```python
from build123d import *

# Parameters (mm, degrees)
SKETCH_1_W           = 270
SKETCH_1_H           = 250
SKETCH_1_R           = 1.55
EXTRUDE_1_DEPTH      = 3
SKETCH_2_R           = 40
CUT_EXTRUDE_1_DEPTH  = 10
CUT_EXTRUDE_3_DEPTH  = 10
SKETCH_5_R           = 5
SKETCH_5_R_2         = 1.55
CUT_EXTRUDE_4_DEPTH  = 10
SKETCH_6_R           = 42.5
CUT_EXTRUDE_5_DEPTH  = 10
SKETCH_8_W           = 100
SKETCH_8_H           = 70
CUT_EXTRUDE_7_DEPTH  = 10
SKETCH_9_R           = 1.55
CUT_EXTRUDE_8_DEPTH  = 10
SKETCH_10_R          = 1.55
CUT_EXTRUDE_9_DEPTH  = 10
SKETCH_11_R          = 1.55
CUT_EXTRUDE_10_DEPTH = 10
FILLET_3_R           = 8
SKETCH_13_W          = 34
SKETCH_13_H          = 48
SKETCH_13_W_2        = 7
SKETCH_13_H_2        = 7
SKETCH_13_R          = 1.55
CUT_EXTRUDE_12_DEPTH = 10
FILLET_4_R           = 1.5
SKETCH_15_R          = 1.55
CUT_EXTRUDE_13_DEPTH = 10
SKETCH_16_R          = 4.05
CUT_EXTRUDE_14_DEPTH = 10
CUT_EXTRUDE_START    = -10
SKETCH_19_R          = 4.05
CUT_EXTRUDE_19_DEPTH = 10
SKETCH_21_R          = 1.55
CUT_EXTRUDE_20_DEPTH = 10
SKETCH_23_W          = 7
SKETCH_23_H          = 19
CUT_EXTRUDE_22_DEPTH = 10
FILLET_8_R           = 2
SKETCH_12_W          = 2
SKETCH_12_H          = 35.6
SKETCH_12_R          = 1.1
CUT_EXTRUDE_23_DEPTH = 10
FILLET_9_R           = 5
SKETCH_26_R          = 1.55
CUT_EXTRUDE_24_DEPTH = 8


with BuildPart() as part:
    # 草图1 → 凸台-拉伸1 (new body)
    with BuildSketch(Plane(origin=(0, 0, 0), x_dir=(1, 0, 0), z_dir=(0, 1, 0))):
        Rectangle(SKETCH_1_W, SKETCH_1_H)
        with Locations(Location((132, 72, 0), (0, 0, 270))):
            Circle(SKETCH_1_R, mode=Mode.SUBTRACT)
        with Locations(Location((132, -72, 0), (0, 0, 270))):
            Circle(SKETCH_1_R, mode=Mode.SUBTRACT)
    extrude(amount=EXTRUDE_1_DEPTH)

    # 草图2 → 切除-拉伸1 (cut)
    with BuildSketch(Plane(origin=(0, 3, 0), x_dir=(1, 0, 0), z_dir=(0, 1, 0))):
        with Locations((-3, -95)):
            Circle(SKETCH_2_R)
    extrude(amount=-CUT_EXTRUDE_1_DEPTH, mode=Mode.SUBTRACT)

    # 草图4 → 切除-拉伸3 (cut)
    with BuildSketch(Plane(origin=(0, 3, 0), x_dir=(1, 0, 0), z_dir=(0, 1, 0))):
        Polygon((-90, -125), (-135, -70), (-162.976707817, -172.035264534), align=None)
        Polygon((-90, 125), (-135, 70), (-171.69806915, 153.777299788), align=None)
    extrude(amount=-CUT_EXTRUDE_3_DEPTH, mode=Mode.SUBTRACT)

    # 草图5 → 切除-拉伸4 (cut)
    with BuildSketch(Plane(origin=(0, 3, 0), x_dir=(1, 0, 0), z_dir=(0, 1, 0))):
        with Locations(Location((-87.852813742, 75, 0), (0, 0, 270))):
            Circle(SKETCH_5_R)
        with Locations(Location((-3, 95, 0), (0, 0, 270))):
            Circle(SKETCH_5_R)
        with Locations(Location((81.852813742, 75, 0), (0, 0, 270))):
            Circle(SKETCH_5_R)
        with Locations(Location((-87.852813742, 90, 0), (0, 0, 270))):
            Circle(SKETCH_5_R_2)
        with Locations(Location((-74.862432686, 67.5, 0), (0, 0, 270))):
            Circle(SKETCH_5_R_2)
        with Locations(Location((-100.843194799, 67.5, 0), (0, 0, 270))):
            Circle(SKETCH_5_R_2)
        with Locations(Location((-3, 110, 0), (0, 0, 270))):
            Circle(SKETCH_5_R_2)
        with Locations(Location((9.990381057, 87.5, 0), (0, 0, 270))):
            Circle(SKETCH_5_R_2)
        with Locations(Location((-15.990381057, 87.5, 0), (0, 0, 270))):
            Circle(SKETCH_5_R_2)
        with Locations(Location((81.852813742, 90, 0), (0, 0, 270))):
            Circle(SKETCH_5_R_2)
        with Locations(Location((94.843194799, 67.5, 0), (0, 0, 270))):
            Circle(SKETCH_5_R_2)
        with Locations(Location((68.862432686, 67.5, 0), (0, 0, 270))):
            Circle(SKETCH_5_R_2)
    extrude(amount=-CUT_EXTRUDE_4_DEPTH, mode=Mode.SUBTRACT)

    # 草图6 → 切除-拉伸5 (cut)
    with BuildSketch(Plane(origin=(0, 3, 0), x_dir=(1, 0, 0), z_dir=(0, 1, 0))):
        with Locations((-3, -95)):
            Circle(SKETCH_6_R)
    extrude(amount=-CUT_EXTRUDE_5_DEPTH, mode=Mode.SUBTRACT)

    # 草图8 → 切除-拉伸7 (cut)
    with BuildSketch(Plane(origin=(0, 3, 0), x_dir=(1, 0, 0), z_dir=(0, 1, 0))):
        with Locations((135, 0)):
            Rectangle(SKETCH_8_W, SKETCH_8_H)
    extrude(amount=-CUT_EXTRUDE_7_DEPTH, mode=Mode.SUBTRACT)

    # 草图9 → 切除-拉伸8 (cut)
    with BuildSketch(Plane(origin=(0, 3, 0), x_dir=(1, 0, 0), z_dir=(0, 1, 0))):
        with Locations(Location((-52.5, 67, 0), (0, 0, 270))):
            Circle(SKETCH_9_R)
    extrude(amount=-CUT_EXTRUDE_8_DEPTH, mode=Mode.SUBTRACT)

    # 草图10 → 切除-拉伸9 (cut)
    with BuildSketch(Plane(origin=(0, 3, 0), x_dir=(1, 0, 0), z_dir=(0, 1, 0))):
        with Locations(Location((57, 103, 0), (0, 0, 270))):
            Circle(SKETCH_10_R)
    extrude(amount=-CUT_EXTRUDE_9_DEPTH, mode=Mode.SUBTRACT)

    # 草图11 → 切除-拉伸10 (cut)
    with BuildSketch(Plane(origin=(0, 3, 0), x_dir=(1, 0, 0), z_dir=(0, 1, 0))):
        with Locations(Location((-52.5, -39, 0), (0, 0, 270))):
            Circle(SKETCH_11_R)
    extrude(amount=-CUT_EXTRUDE_10_DEPTH, mode=Mode.SUBTRACT)

    # 圆角3
    fillet_3_edges = [part.edges().sort_by_distance(p)[0] for p in [
        (135, 1.5, 35),
        (135, 1.5, -35),
        (85, 1.5, 35),
        (85, 1.5, -35),
        (-135, 1.5, -70),
        (-135, 1.5, 70),
        (-90, 1.5, -125),
        (135, 1.5, 125),
        (135, 1.5, -125),
    ]]
    fillet(fillet_3_edges, radius=FILLET_3_R)

    # 草图13 → 切除-拉伸12 (cut)
    with BuildSketch(Plane(origin=(0, 3, 0), x_dir=(1, 0, 0), z_dir=(0, 1, 0))):
        with Locations((10, 26)):
            Rectangle(SKETCH_13_W, SKETCH_13_H)
        with Locations((30.5, 26)):
            Rectangle(SKETCH_13_W_2, SKETCH_13_H)
        with Locations((10, 53.5)):
            Rectangle(SKETCH_13_W, SKETCH_13_H_2)
        with Locations((-10.5, 26)):
            Rectangle(SKETCH_13_W_2, SKETCH_13_H)
        with Locations((10, -1.5)):
            Rectangle(SKETCH_13_W, SKETCH_13_H_2)
        with Locations(Location((30, 0, 0), (0, 0, 270))):
            Circle(SKETCH_13_R)
        with Locations(Location((-10, 52, 0), (0, 0, 270))):
            Circle(SKETCH_13_R)
        with Locations(Location((-10, 0, 0), (0, 0, 270))):
            Circle(SKETCH_13_R)
        with Locations(Location((30, 52, 0), (0, 0, 270))):
            Circle(SKETCH_13_R)
    extrude(amount=-CUT_EXTRUDE_12_DEPTH, mode=Mode.SUBTRACT)

    # 圆角4
    fillet_4_edges = [part.edges().sort_by_distance(p)[0] for p in [
        (-7, 1.5, -2),
        (-14, 1.5, -2),
        (-14, 1.5, -50),
        (-7, 1.5, -50),
        (-7, 1.5, -57),
        (27, 1.5, -57),
        (27, 1.5, -50),
        (34, 1.5, -50),
        (34, 1.5, -2),
        (27, 1.5, -2),
        (27, 1.5, 5),
        (-7, 1.5, 5),
    ]]
    fillet(fillet_4_edges, radius=FILLET_4_R)

    # 草图15 → 切除-拉伸13 (cut)
    with BuildSketch(Plane(origin=(0, 3, 0), x_dir=(1, 0, 0), z_dir=(0, 1, 0))):
        with Locations(Location((47.5, -105, 0), (0, 0, 270))):
            Circle(SKETCH_15_R)
        with Locations(Location((-52.5, -105, 0), (0, 0, 270))):
            Circle(SKETCH_15_R)
        with Locations(Location((47.5, -57, 0), (0, 0, 270))):
            Circle(SKETCH_15_R)
        with Locations(Location((-52.5, -57, 0), (0, 0, 270))):
            Circle(SKETCH_15_R)
    extrude(amount=-CUT_EXTRUDE_13_DEPTH, mode=Mode.SUBTRACT)

    # 草图16 → 切除-拉伸14 (cut)
    with BuildSketch(Plane.XZ):
        with Locations(Location((-53, -105, 0), (0, 0, 270))):
            Circle(SKETCH_16_R)
    extrude(amount=-CUT_EXTRUDE_14_DEPTH, mode=Mode.SUBTRACT)

    # 草图19 → 切除-拉伸19 (cut)
    with BuildSketch(Plane(origin=(0, 3, 0), x_dir=(1, 0, 0), z_dir=(0, 1, 0)).offset(CUT_EXTRUDE_START)):
        with Locations(Location((-53, 105, 0), (0, 0, 90))):
            Circle(SKETCH_19_R)
        with Locations(Location((47, 105, 0), (0, 0, 270))):
            Circle(SKETCH_19_R)
    extrude(amount=CUT_EXTRUDE_19_DEPTH, mode=Mode.SUBTRACT)

    # 草图21 → 切除-拉伸20 (cut)
    with BuildSketch(Plane(origin=(0, 0, 0), x_dir=(-1, 0, 0), z_dir=(0, -1, 0))):
        with Locations(Location((-132.26, -117.45, 0), (0, 0, 90))):
            Circle(SKETCH_21_R)
        with Locations(Location((-70.88, -117.45, 0), (0, 0, 90))):
            Circle(SKETCH_21_R)
        with Locations(Location((-70.88, -81.94, 0), (0, 0, 90))):
            Circle(SKETCH_21_R)
        with Locations(Location((-132.26, -81.94, 0), (0, 0, 90))):
            Circle(SKETCH_21_R)
    extrude(amount=-CUT_EXTRUDE_20_DEPTH, mode=Mode.SUBTRACT)

    # 草图23 → 切除-拉伸22 (cut)
    with BuildSketch(Plane(origin=(0, 0, 0), x_dir=(-1, 0, 0), z_dir=(0, -1, 0))):
        with Locations((-131.5, -94.44)):
            Rectangle(SKETCH_23_W, SKETCH_23_H)
    extrude(amount=-CUT_EXTRUDE_22_DEPTH, mode=Mode.SUBTRACT)

    # 圆角8
    fillet_8_edges = [part.edges().sort_by_distance(p)[0] for p in [
        (135, 1.5, 103.94),
        (135, 1.5, 84.94),
        (128, 1.5, 84.94),
        (128, 1.5, 103.94),
    ]]
    fillet(fillet_8_edges, radius=FILLET_8_R)

    # 草图12 → 切除-拉伸23 (cut)
    with BuildSketch(Plane(origin=(0, 3, 0), x_dir=(1, 0, 0), z_dir=(0, 1, 0))):
        with Locations((-113.775, 0)):
            Rectangle(SKETCH_12_W, SKETCH_12_H)
        with Locations((-111.775, 0)):
            Rectangle(SKETCH_12_W, SKETCH_12_H)
        Polygon((-73.975, 31.25), (-112.775, 31.25), (-112.775, 17.8), (-110.775, 17.8), (-110.775, -17.8), (-112.775, -17.8), (-112.775, -31.25), (-73.975, -31.25), align=None)
        with Locations(Location((-112.975, 34.2, 0), (0, 0, 270))):
            Circle(SKETCH_12_R)
        with Locations(Location((-73.975, 34.2, 0), (0, 0, 270))):
            Circle(SKETCH_12_R)
        with Locations(Location((-112.975, -34.2, 0), (0, 0, 270))):
            Circle(SKETCH_12_R)
        with Locations(Location((-73.975, -34.2, 0), (0, 0, 270))):
            Circle(SKETCH_12_R)
    extrude(amount=-CUT_EXTRUDE_23_DEPTH, mode=Mode.SUBTRACT)

    # 圆角9
    fillet_9_edges = [part.edges().sort_by_distance(p)[0] for p in [
        (27.103986447, 1.5, 125),
        (-33.103986447, 1.5, 125),
    ]]
    fillet(fillet_9_edges, radius=FILLET_9_R)

    # 草图26 → 切除-拉伸24 (cut)
    with BuildSketch(Plane(origin=(0, 0, 0), x_dir=(-1, 0, 0), z_dir=(0, -1, 0))):
        with Locations(Location((-132.26, -106.94, 0), (0, 0, 90))):
            Circle(SKETCH_26_R)
        with Locations(Location((-70.88, -106.94, 0), (0, 0, 90))):
            Circle(SKETCH_26_R)
    extrude(amount=-CUT_EXTRUDE_24_DEPTH, mode=Mode.SUBTRACT)


solid = part.part
```
Verification items for the finished model (mm, model axes). A direction names the side the tool comes from. Give positions to 0.01 mm unless a question says otherwise; leave off trailing zeros. Order: outer loops, then holes, each group sorted by start corner. A loop starts at its lowest first (then second) coordinate and runs counter-clockwise, first axis right, second up. Notation, with made-up numbers: (38, 23) - (76, 23) arc R4 ccw to (76, 28) - close; hole circle Ø11 at (-30, 12.25). An arc over 180 degrees is marked (long way). Answer as CSV lines item,"result". Start each with the question number.
Item 1: Section check B-B, the plane y = 2.25. State how many separate pieces and enclosed holes the cut face has, plus the area to 3 significant figures.
Item 2: Mould release check, pull along Z, two halves, no side actions. Record for faces 1 (the face through (-112.5, 1.5, -97.5)), 2 (the face through (-32, 0, -2)), 3 (the face through (77.42, 1.52, -72.69)), 4 (the face through (-4.915, 1.521, -90.381)): released by +Z, released by -Z, zero draft, split by the parting line, or undercut.
Item 3: Material ranges on L1, parallel to X at y = 2.6, z = -8 (3 decimals); L2, parallel to X at y = 0.25, z = -48.5; L3, parallel to X at y = 2.45, z = -67, recorded low to high.
Item 4: Access from +Z, -Z, +X, -X, +Y, -Y to the whole of each face (thin tool, end or side, straight path). Record for faces 5 (the face through (132.594, 1.521, 122.719)), 6 (the face through (87.406, 1.479, -32.719)).
Item 5: Section check A-A, the plane z = 95. Record the boundary of the cut face in (x, y), plus the area to 3 significant figures.
Item 6: Gauge pin test, flat end, axial feed: pin 1 (3.5 mm diameter, centred on x = 70.88, z = 106.94, fed in from -Y). Record the tip position at first contact, or that the pin passes through.
Filled in:
1,separate pieces,"1"
1,enclosed holes,"39"
1,area,"50,300 mm^2"
2,face 1,"released by -Z"
2,face 2,"zero draft"
2,face 3,"undercut"
2,face 4,"undercut"
3,L1,"-135 to -114.775, -73.975 to -14, 34 to 85"
3,L2,"-135 to -14, 34 to 135"
3,L3,"-135 to -102.31, -99.38 to -76.33, -73.4 to -54.05, -50.95 to 67.4, 70.33 to 93.38, 96.31 to 135"
4,face 5,"+Z, +X, +Y, -Y"
4,face 6,"+X, +Y, -Y"
5,outline,"(-114.55, 0) - (-45.5, 0) - (-45.5, 3) - (-114.55, 3) - close; (39.5, 0) - (128, 0) - (128, 3) - (39.5, 3) - close"
5,area,"473 mm^2"
6,pin 1,"y = 0"
